Geometry check sheet. Reference: the model listing, model coordinates, mm. A direction names the side the tool comes from. Coordinates: 2 decimals unless noted, no trailing zeros. Loops run counter-clockwise (first coordinate to the right, second up) from the corner with the lowest first, then second, coordinate; pieces in that order, holes last. Notation, with made-up numbers: M 38,47 L 49,47 A19 ccw 49,76 Z; hole C 18.25,-11 d11. An arc over 180 degrees is marked long. Use CSV: the item, a comma, the result in double quotes.
```python
from build123d import *

# Parameters (mm, degrees)
SKETCH1_R           = 10
BOSS_EXTRUDE1_DEPTH = 20
BOSS_EXTRUDE2_REACH = 205.079
CUT_EXTRUDE1_REACH  = 215.698
SKETCH3_R           = 15


with BuildPart() as part:
    # Sketch1 → Boss-Extrude1 (new body)
    with BuildSketch(Plane(origin=(0, 0, 0), x_dir=(1, 0, 0), z_dir=(0, 1, 0))):
        with BuildLine():
            Line((0, 51), (0, -51))
            ThreePointArc((0, -51), (20, -71), (40, -51))
            Line((40, -51), (40, -30))
            Line((40, -30), (170, -30))
            ThreePointArc((170, -30), (177.071067812, -27.071067812), (180, -20))
            Line((180, -20), (180, -10))
            Line((180, -10), (160, -10))
            ThreePointArc((160, -10), (150, 0), (160, 10))
            Line((160, 10), (180, 10))
            Line((180, 10), (180, 20))
            ThreePointArc((180, 20), (177.071067812, 27.071067812), (170, 30))
            Line((170, 30), (40, 30))
            Line((40, 30), (40, 51))
            ThreePointArc((40, 51), (20, 71), (0, 51))
        make_face()
        with Locations(Location((20, -51, 0), (0, 0, 270))):
            Circle(SKETCH1_R, mode=Mode.SUBTRACT)
        with Locations(Location((20, 51, 0), (0, 0, 90))):
            Circle(SKETCH1_R, mode=Mode.SUBTRACT)
    extrude(amount=BOSS_EXTRUDE1_DEPTH)

    # Boss-Extrude2: up to this face of the body (flat: up to its plane)
    boss_extrude2_end = Plane(part.part.faces().sort_by_distance((73.396795742, 20, 0))[0])
    # Sketch2 → Boss-Extrude2 (add, up to the picked face)
    with BuildSketch(Plane(origin=(-10, 10, 0), x_dir=(0, 0, 1), z_dir=(-0.7071067811865512, 0.7071067811865438, 0)), mode=Mode.PRIVATE) as boss_extrude2_sk1:
        with BuildLine():
            Line((30, 14.142135624), (-30, 14.142135624))
            Line((-30, 14.142135624), (-30, 65.142135624))
            ThreePointArc((-30, 65.142135624), (0, 95.142135624), (30, 65.142135624))
            Line((30, 65.142135624), (30, 14.142135624))
        make_face()
    boss_extrude2_tool1 = split(extrude(boss_extrude2_sk1.sketch, amount=-BOSS_EXTRUDE2_REACH, mode=Mode.PRIVATE), bisect_by=boss_extrude2_end, keep=Keep.BOTH, mode=Mode.PRIVATE)
    add(boss_extrude2_tool1.solids().sort_by(Axis((26.574223, 46.574223, 0), (0.7071067811865512, -0.7071067811865438, 0)))[0])

    # Cut-Extrude1: up to this plane
    cut_extrude1_end = Plane(origin=(20, 0, 51), z_dir=(0, 1, 0))
    # Sketch3 → Cut-Extrude1 (cut, up to the surface)
    with BuildSketch(Plane(origin=(-10, 10, 0), x_dir=(0, 0, 1), z_dir=(-0.7071067811865513, 0.7071067811865438, 0)), mode=Mode.PRIVATE) as cut_extrude1_sk1:
        with Locations(Location((0, 65.142135624, 0), (0, 0, 270))):
            Circle(SKETCH3_R)
    cut_extrude1_tool1 = split(extrude(cut_extrude1_sk1.sketch, amount=-CUT_EXTRUDE1_REACH, mode=Mode.PRIVATE), bisect_by=cut_extrude1_end, keep=Keep.BOTH, mode=Mode.PRIVATE)
    add(cut_extrude1_tool1.solids().sort_by_distance((36.062446, 56.062446, 0))[0], mode=Mode.SUBTRACT)


solid = part.part
```
1. Section check C-C, the plane x = 137.5. Record the cut outline in (y, z).
The answers:
outline,"M 0,-30 L 20,-30 L 20,30 L 0,30 Z"
2. Set-up check for faces 1 (the flat face through (170, 10, 10)), 2 (the flat face through (40, 10, 41)), 3 (the flat face through (40, 10, -40)): record each of +Z, -Z, +X, -X, +Y, -Y from which the full face is reachable in a straight line by a thin tool's end or side.
The answers:
face 1,"+X, +Y, -Y"
face 2,"+Z, +X, +Y, -Y"
face 3,"-Z, +X, +Y, -Y"
3. Release check for a two-part mould opening along X. For faces 4 (the cylindrical face through (72.29, 41.03, 0.66)), 5 (the flat face through (24.2, 20, -41.7)), 6 (the cylindrical face through (20, 10, 71)), 7 (the flat face through (0, 10, -1)) record: +X half, -X half, draft (parallel to the pull), parting line (faces both ways), or undercut.
The answers:
face 4,"undercut"
face 5,"draft"
face 6,"parting line"
face 7,"-X half"
4. Section check B-B, the plane z = -2.5. Record the cut outline in (x, y), plus the area to 3 significant figures.
The answers:
outline,"M 0,0 L 71.21,0 L 25.6,45.6 L 0,20 Z; M 46.52,66.52 L 113.04,0 L 150.32,0 L 150.32,20 L 114.4,20 L 57.2,77.2 Z"
area,"3,930 mm^2"
5. Section check A-A, the plane x = 20. Record the cut outline in (y, z).
The answers:
outline,"M 0,-71 L 20,-71 L 20,-61 L 0,-61 Z; M 0,-41 L 20,-41 L 20,-30 L 40,-30 L 40,30 L 20,30 L 20,41 L 0,41 Z; M 0,61 L 20,61 L 20,71 L 0,71 Z"
6. Section check D-D, the plane z = 27.5. Record the cut outline in (x, y), plus the area to 3 significant figures.
The answers:
outline,"M 0,0 L 176.61,0 L 176.61,20 L 89.08,20 L 44.54,64.54 L 0,20 Z"
area,"5,520 mm^2"
7. Thickness scan on line 1 (X direction, y = 6.75, z = 51); line 2 (Y direction, x = 10, z = 39.5); line 3 (Z direction, x = 152.5, y = 14.5). Record the ranges inside material, lowest first. Write a range as [from, to].
The answers:
line 1,"[0, 10], [30, 40]"
line 2,"[0, 20]"
line 3,"[-30, -6.61], [6.61, 30]"
8. Gauge pin test, flat ends, axial feed: P1, Ø6, axis at y = 39, z = -20.5, coming from the +X side; P2, Ø6, axis at x = 174.5, y = 7, coming from the -Z side; P3, Ø22, axis at y = 6, z = 41.5, coming from the +X side. Record the tip position at first contact, or that the pin passes through.
The answers:
P1,"x = 88.78"
P2,"z = -29.89"
P3,"x = 40"
